Read the model definition and answer for the solid it produces. Units are mm, in the model's axes. A direction names the side the tool comes from. Coordinates: 2 decimals unless noted, no trailing zeros. Write each loop counter-clockwise with the first axis right and the second up, starting at its lowest first coordinate (ties: lowest second). Pieces come first, ordered by that corner, then holes.
Item 1: Section C-C (x = 249.5) is taken. Give the vertices of the cut face in (y, z), then the cut area to 3 significant figures.
Item 2: Section A-A (x = 433) is taken. Give the vertices of the cut face in (y, z).
Item 3: Section D-D (z = 1.55) is taken. Give the vertices of the cut face in (x, y), then the cut area to 3 significant figures.
Item 4: Section B-B (y = 889) is taken. Give the vertices of the cut face in (x, z), then the cut area to 4 significant figures.
Item 5: Each of these flat-tipped pins is pushed along its axis until it touches: P1, Ø0.8, axis at x = 352, z = 1.5, coming from the +Y side; P2, Ø1.3, axis at y = 450, z = 1.5, coming from the +X side; P3, Ø0.8, axis at x = 398, z = 1.5, coming from the +Y side. Where does it stop, or does it pass through?
Item 6: Determine the mould class of faces 1 (the face through (319.728, 581.903, 1.252)), 2 (the face through (278.749, 507.344, 1.252)), 3 (the face through (537.622, 986.758, 1.252)), 4 (the face through (390, 700, 0)) for opening direction Y: released by +Y, released by -Y, zero draft, split by the parting line, or undercut.
Item 7: A tool of negligible diameter and unlimited length cuts with its end or side. For faces 5 (the face through (282.126, 501.654, 1.252)), 6 (the face through (390, 700, 2.54)), from which of +Z, -Z, +X, -X, +Y, -Y can it reach the whole face along a straight path? Write none if from no direction.
Item 8: Straight lines are drawn through the part: probe 1 along Y at (x, z) = (381.5, 0.4); probe 2 along Y at (x, z) = (308, 1.55); probe 3 along X at (y, z) = (477, 0.35). For each, find the intervals that lie inside material, in ascending order.
Autodesk Inventor part; units mm, degrees
ref_plane "YZ Plane" through (0, 0, 0) normal (1, 0, 0) x (0, 1, 0)
ref_plane "XZ Plane" through (0, 0, 0) normal (0, 1, 0) x (-1, 0, 0)
ref_plane "XY Plane" through (0, 0, 0) normal (0, 0, 1) x (1, 0, 0)
sketch "Sketch1" plane through (0, 0, 0) normal (0, 0, 1) x (1, 0, 0)
  arc A0 (368.3, 596.9) -> (621.266, 1035.05) centre (368.3, 889) ccw
  circle A1 centre (368.3, 889) radius 101.6
  line L0 (621.266, 1035.05) -> (368.3, 889) construction
  line L1 (456.2882, 939.8) -> (14.5272, 1704.9525) construction
  line L2 (456.2882, 939.8) -> (-427.2338, 939.8) construction
  line L3 (368.3, 889) -> (368.3, 596.9) construction
  line L4 (368.3, 596.9) -> (342.9, 596.9)
  line L5 (342.9, 596.9) -> (342.9, 787.4) construction
  line L6 (342.9, 787.4) -> (368.3, 787.4)
  line L7 (0, 0) -> (685.8, 0) construction
  line L8 (685.8, 0) -> (685.8, 1498.6) construction
  line L9 (685.8, 1498.6) -> (0, 1498.6) construction
  line L10 (0, 1498.6) -> (0, 0) construction
  line L11 (241.3, 0) -> (444.5, 0) construction
  line L12 (444.5, 0) -> (444.5, 558.8) construction
  line L13 (444.5, 558.8) -> (241.3, 558.8) construction
  line L14 (241.3, 558.8) -> (241.3, 0) construction
  line L15 (241.3, 135.2277) -> (0, 135.2277) construction
  line L16 (444.5, 135.2277) -> (685.8, 135.2277) construction
  line L17 (456.2882, 939.8) -> (621.266, 1035.05)
  arc A2 (342.9, 596.9) -> (342.9, 546.1) centre (342.9, 571.5) ccw
  arc A3 (342.9, 787.4) -> (342.9, 355.6) centre (342.9, 571.5) ccw
  line L18 (342.9, 546.1) -> (444.5, 546.1)
  line L19 (342.9, 355.6) -> (444.5, 355.6)
  line L20 (444.5, 355.6) -> (444.5, 546.1)
  arc A4 (342.9, 787.4) -> (343.2908, 790.5262) centre (342.9, 788.9875) ccw
  circle A5 centre (342.9, 571.5) radius 25.4
  line L21 (323.3933, 555.232) -> (232.8369, 458.0957)
  line L22 (237.4816, 453.7656) -> (232.8369, 458.0957)
  line L23 (237.4816, 453.7656) -> (328.038, 550.9019)
  line L24 (328.038, 550.9019) -> (323.3933, 555.232)
  line L25 (357.762, 592.0981) -> (448.3184, 689.2344)
  line L26 (448.3184, 689.2344) -> (452.9631, 684.9043)
  line L27 (452.9631, 684.9043) -> (362.4067, 587.768)
  line L28 (362.4067, 587.768) -> (357.762, 592.0981)
  dimension "d0" = 203.2
  dimension "d2" = 60
  dimension "d3" = 120
  dimension "d5" = 685.8
  dimension "d6" = 1498.6
  dimension "d7" = 203.2
  dimension "d8" = 558.8
  dimension "d9" = 190.5
  dimension "d14" = 25.4
  dimension "d15" = 939.8
  dimension "d21" = 25.4
  dimension "d22" = 101.6
  dimension "d25" = 6.35
extrude "Extrusion2" add sketch "Sketch1" along normal blind 2.54 contours L4 L25 L26 L27 A0 | L27 L26 L25 L4 A2 L21 L22 L23 L18 L20 L19 A3 L6 A1 L17 A0 | A1
properties part number "ShooterSketch"
Established:
1. outline: (376.85, 0) - (466.66, 0) - (466.66, 2.54) - (376.85, 2.54) - close; (475.97, 0) - (766.15, 0) - (766.15, 2.54) - (475.97, 2.54) - close
1. area: 965 mm2
2. outline: (355.6, 0) - (546.1, 0) - (546.1, 2.54) - (355.6, 2.54) - close; (604.16, 0) - (967.34, 0) - (967.34, 2.54) - (604.16, 2.54) - close
3. outline: (232.84, 458.1) - (323.39, 555.23) arc R25.4 cw to (342.9, 596.9) - (368.3, 596.9) arc R292.1 ccw to (621.27, 1035.05) - (456.29, 939.8) arc R101.6 ccw (long way) to (368.3, 787.4) - (342.9, 787.4) arc R215.9 ccw to (342.9, 355.6) - (444.5, 355.6) - (444.5, 546.1) - (342.9, 546.1) arc R25.4 cw to (328.04, 550.9) - (237.48, 453.77) - close
3. area: 207,000 mm2
4. outline: (266.7, 0) - (660.4, 0) - (660.4, 2.54) - (266.7, 2.54) - close
4. area: 1,000 mm2
5. P1: stops at y = 989.35
5. P2: stops at x = 444.5
5. P3: stops at y = 986.28
6. face 1: undercut
6. face 2: undercut
6. face 3: released by +Y
6. face 4: zero draft
7. face 5: +Z, -Z
7. face 6: +Z, +X, -X, +Y, -Y
8. probe 1: y = 355.6 to 546.1, 597.2 to 989.74
8. probe 2: y = 358.44 to 529.41, 538.72 to 784.56, 807.23 to 970.77
8. probe 3: x = 148.78 to 250.46, 259.14 to 444.5
